Check sheet for the drawn part. Datum: minimum x, y, z corner. Units: mm. Round coordinates to 2 decimals unless told otherwise and drop trailing zeros. Write each loop counter-clockwise with the first axis right and the second up, starting at its lowest first coordinate (ties: lowest second). Pieces come first, ordered by that corner, then holes.
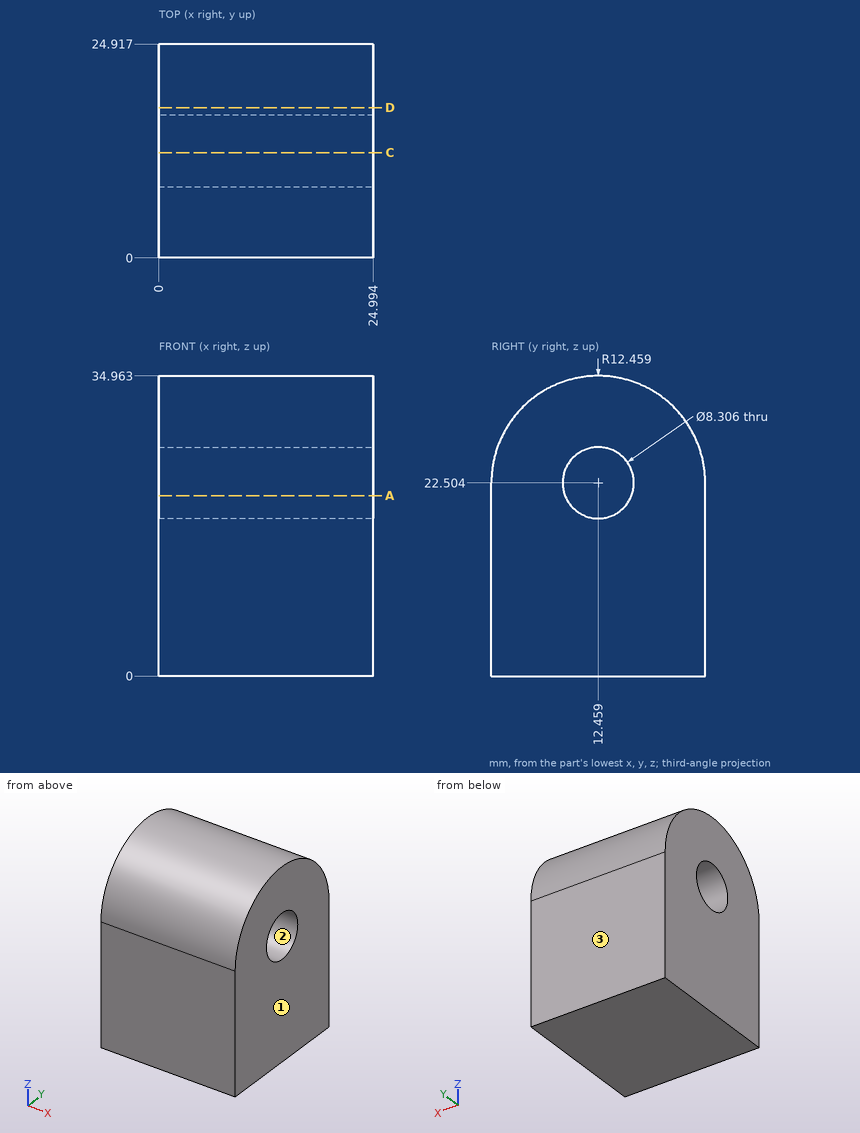
1. Release check for a two-part mould opening along Y. For the marked faces 1, 2 and 3 record: released by +Y, released by -Y, zero draft, split by the parting line, or undercut.
2. Scan lines: line 1 along Y through (x, z) = (2, 22.5) (1 decimal); line 2 along Z through (x, y) = (2.75, 15.25) (1 decimal); line 3 along Z through (x, y) = (6.25, 15.75) (1 decimal). Record each from-to range of solid material in increasing order.
3. Sectioned sample at A-A, the plane z = 21. Enter the section's corners in (x, y), plus the area to 3 significant figures.
4. Sectioned sample at C-C, the plane y = 12.25. Enter the section's corners in (x, z).
5. Go/stop test with flat-tipped pins: pin 1 (5 mm diameter, centred on x = 8, y = 6, fed in from +Z); pin 2 (5 mm diameter, centred on x = 9, y = 22, fed in from +Z); pin 3 (12 mm diameter, centred on x = 22.5, y = 19, fed in from +Z). Record where each tip stops, or that it passes through.
6. Sectioned sample at D-D, the plane y = 17.5. Enter the section's corners in (x, z).
Computed values:
1. face 1: zero draft
1. face 2: undercut
1. face 3: released by +Y
2. line 1: y = 0 to 8.3, 16.6 to 24.9
2. line 2: z = 0 to 19.4, 25.6 to 34.6
2. line 3: z = 0 to 20, 25 to 34.5
3. outline: (0, 0) - (24.99, 0) - (24.99, 8.59) - (0, 8.59) - close; (0, 16.33) - (24.99, 16.33) - (24.99, 24.92) - (0, 24.92) - close
3. area: 429 mm2
4. outline: (0, 0) - (24.99, 0) - (24.99, 18.36) - (0, 18.36) - close; (0, 26.65) - (24.99, 26.65) - (24.99, 34.96) - (0, 34.96) - close
5. pin 1: stops at z = 34.32
5. pin 2: stops at z = 32.78
5. pin 3: stops at z = 34.95
6. outline: (0, 0) - (24.99, 0) - (24.99, 33.9) - (0, 33.9) - close
